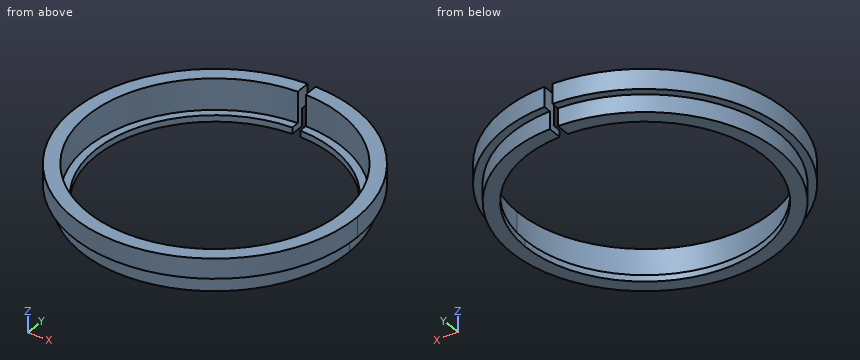
Autodesk Inventor part; units mm, degrees
ref_plane "YZ Plane" through (0, 0, 0) normal (1, 0, 0) x (0, 1, 0)
ref_plane "XZ Plane" through (0, 0, 0) normal (0, 1, 0) x (-1, 0, 0)
ref_plane "XY Plane" through (0, 0, 0) normal (0, 0, 1) x (1, 0, 0)
sketch "Sketch1" plane through (0, 0, 0) normal (0, 0, 1) x (1, 0, 0)
  circle A0 centre (0, 0) radius 16.8
  circle A1 centre (0, 0) radius 15
  circle A2 centre (0, 0) radius 17.8
  circle A3 centre (0, 0) radius 16
  dimension "d0" = 33.6
  dimension "d1" = 30
  dimension "d2" = 35.6
  dimension "d3" = 32
extrude "Extrusion1" add sketch "Sketch1" along normal blind 0.8 contours A3
extrude "Extrusion2" add sketch "Sketch1" along normal blind 3.2 contours A0
sketch "Sketch2" plane through (0, 0, 3.2) normal (0, 0, 1) x (1, 0, 0)
  circle A0 centre (0, 0) radius 17.8
  circle A1 centre (0, 0) radius 16
extrude "Extrusion3" add sketch "Sketch2" along normal blind 1.5
extrude "Extrusion5" add sketch "Sketch2" against normal blind 1
sketch "Sketch3" plane through (0, 0, 4.7) normal (0, 0, 1) x (1, 0, 0)
  line L0 (0.5, 8) -> (-0.5, 8)
  line L1 (-0.5, 8) -> (-0.5, 24)
  line L2 (-0.5, 24) -> (0.5, 24)
  line L3 (0.5, 24) -> (0.5, 8)
  circle A0 centre (0, 0) radius 16
  line L4 (0.5, 8) -> (-0.5, 24) construction
  line L5 (-0.5, 8) -> (0.5, 24) construction
  point P0 (0, 16)
  dimension "d10" = 1
  dimension "d11" = 16
extrude "Extrusion4" cut sketch "Sketch3" against normal blind 10 contours L0 L1 A0 L3 | A0 L1 L2 L3 picked at (0.0556, 10.6664)
properties part number "32to36mm-FilterAdapter"
Build history of the part. All positions in model axes, mm. Give positions to 0.01 mm unless a question says otherwise; leave off trailing zeros. Order: outer loops, then holes, each group sorted by start corner. A loop starts at its lowest first (then second) coordinate and runs counter-clockwise, first axis right, second up. Notation, with made-up numbers: M 13,-14 L 71,-14 A27 ccw 71,10 Z; hole C 82,41 d2. An arc over 180 degrees is marked long. Write item = value, one per line. Start each with the question number.
(1) Probe L1, parallel to Y at x = 0, z = 2.05; L2, parallel to Y at x = 0, z = 2.6; L3, parallel to Z at x = -11.5, y = 13. List the from-to ranges inside material, lowest first. Write a range as [from, to].
(2) Pin check, flat tips, straight feed: pin 1 Ø2 at (x, z) = (-12, 4) entering from -Y; pin 2 Ø1.4 at (y, z) = (16.5, 3.5) entering from -X; pin 3 Ø2 at (x, y) = (-9, 11.5) entering from -Z; pin 4 Ø6 at (x, y) = (7.5, -9.5) entering from +Z. Stop position of each tip, or through.
(3) Slice it at A-A on x = 1. Write the cut outline in (y, z).
(4) Slice it at D-D on z = 3.35. Write the cut outline in (x, y).
(5) Slice it at B-B on y = -5.5. Write the cut outline in (x, z), plus the area to 3 significant figures.
(6) Slice it at C-C on z = 1.4. Write the cut outline in (x, y).
Responses:
q1.L1 = [-16.8, -16]
q1.L2 = [-17.8, -16]
q1.L3 = [2.2, 4.7]
q2.pin_1 = -13.99
q2.pin_2 = -8.2
q2.pin_3 = 0
q2.pin_4 = 0.8
q3.outline = M -17.77,2.2 L -16.77,2.2 L -16.77,0 L -14.97,0 L -14.97,0.8 L -15.97,0.8 L -15.97,4.7 L -17.77,4.7 Z; M 14.97,0 L 16.77,0 L 16.77,2.2 L 17.77,2.2 L 17.77,4.7 L 15.97,4.7 L 15.97,0.8 L 14.97,0.8 Z
q4.outline = M -0.5,15.99 L -0.5,17.79 A17.8 ccw long 0.5,17.79 L 0.5,15.99 A16 cw long Z
q5.outline = M -16.93,2.2 L -15.87,2.2 L -15.87,0 L -13.96,0 L -13.96,0.8 L -15.02,0.8 L -15.02,4.7 L -16.93,4.7 Z; M 13.96,0 L 15.87,0 L 15.87,2.2 L 16.93,2.2 L 16.93,4.7 L 15.02,4.7 L 15.02,0.8 L 13.96,0.8 Z
q5.area = 15.0 mm2
q6.outline = M -0.5,15.99 L -0.5,16.79 A16.8 ccw long 0.5,16.79 L 0.5,15.99 A16 cw long Z
